Could you check a few things on this model? Use its own coordinates, in mm. Face numbers are marked on the shaded views. A direction names the side the tool comes from. Round coordinates to 2 decimals unless told otherwise and drop trailing zeros. Loops run counter-clockwise (first coordinate to the right, second up) from the corner with the lowest first, then second, coordinate; pieces in that order, holes last. Notation, with made-up numbers: (64.25, 46.25) - (87.25, 46.25) arc R17 ccw to (87.25, 61.25) - close; hole circle Ø7 at (2.25, 12.25). An arc over 180 degrees is marked (long way). Use one line per item in the form item = value.
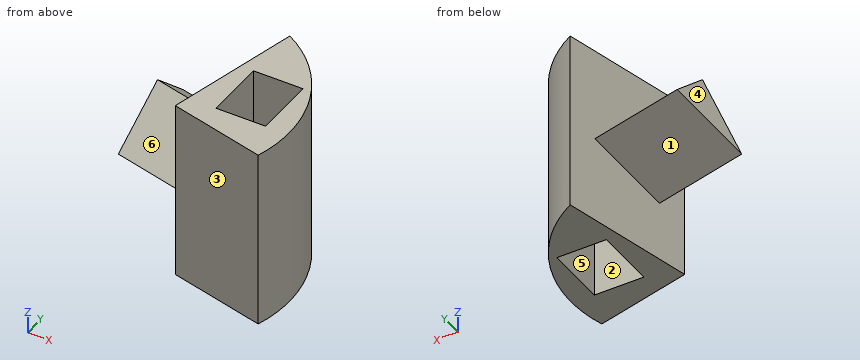
```python
from build123d import *

# Parameters (mm, degrees)
F0_W     = 12.7
F0_H     = 15.9213780425
F1_DEPTH = 46.482
F3_DEPTH = 25.4


with BuildPart() as f1:
    # F0 (on Top) → F1 (new body)
    with BuildSketch(Plane.XY):
        with BuildLine():
            ThreePointArc((16.7416256447, -20.4212910858), (15.8982302722, 2.9417746338), (0.3078590999, 20.3625806509))
            Line((0.3078590999, 20.3625806509), (-8.168171327, -14.3365160608))
            Line((-8.168171327, -14.3365160608), (16.7416256447, -20.4212910858))
        make_face()
        with Locations((6.35, -2.5750233326)):
            Rectangle(F0_W, F0_H, mode=Mode.SUBTRACT)
    extrude(amount=F1_DEPTH)

    # F2 (on face) → F3 (join)
    with BuildSketch(Plane(origin=(-4.40340964, 1.0756312881, 0), x_dir=(-0.2372953486, -0.9714375521, 0), z_dir=(-0.9714375521, 0.2372953486, 0))):
        Polygon((8.0335900158, 15.4112059095), (-4.2063454166, 29.3332058936), (-12.0916292071, 22.4006269127), align=None)
    extrude(amount=F3_DEPTH)


solid = f1.part
```
1. Please list where these lines run through material, in increasing order: line 1 along Y through (x, z) = (7.5, 20.5); line 2 along X through (y, z) = (3, 4); line 3 along X through (y, z) = (-3, 37).
Solution:
line_1 = -18.16 to -10.54, 5.39 to 15.2
line_2 = -3.93 to 0, 12.7 to 15.87
line_3 = -5.4 to 0, 12.7 to 17.69
2. If we section it at C-C, the plane y = 15.5: Write out the boundary of the cut face in (x, z).
Solution:
outline = (-27.03, 21.2) - (-12.5, 22.4) - (-27.03, 25.43) - close; (-0.88, 0) - (7.17, 0) - (7.17, 46.48) - (-0.88, 46.48) - close
3. For P1, Ø5, axis at x = -10, z = 27.5, coming from the +Y side; P2, Ø2, axis at x = -0.5, z = 9.5, coming from the -Y side; P3, Ø6.5, axis at x = 4.5, z = 27, coming from the -Y side, each with a flat end and sliding along its axis, tell me the tip position at first contact or that it passes through.
Solution:
P1 = 11.91
P2 = -16.45
P3 = -18.22
4. On a 3-axis mill with a long thin cutter (end or side, diameter ignored), from which of +Z, -Z, +X, -X, +Y, -Y can I reach the whole of each face in a straight line? I mean the marked faces 4, 5 and 6. Say none if no direction works.
Solution:
face_4 = +Z, -Z, -X, +Y
face_5 = +Z, -Z
face_6 = +Z, -X
5. If we section it at A-A, the plane z = 7: Write out the boundary of the cut face in (x, y).
Solution:
outline = (-8.17, -14.34) - (16.74, -20.42) arc R34.38 ccw to (0.31, 20.36) - close; hole (0, -10.54) - (12.7, -10.54) - (12.7, 5.39) - (0, 5.39) - close
6. If we section it at B-B, the plane x = 10: Write out the boundary of the cut face in (y, z), plus the area to 3 significant figures.
Solution:
outline = (-18.77, 0) - (-10.54, 0) - (-10.54, 46.48) - (-18.77, 46.48) - close; (5.39, 0) - (12.6, 0) - (12.6, 46.48) - (5.39, 46.48) - close
area = 718 mm^2
7. We'd pull the mould along Y, two halves only. Please class the marked faces 1, 2 and 3: +Y half, -Y half, draft (parallel to the pull), parting line (faces both ways), or undercut.
Solution:
face_1 = +Y half
face_2 = undercut
face_3 = -Y half
8. If we section it at D-D, the plane y = 7.5: Write out the boundary of the cut face in (x, z), plus the area to 3 significant figures.
Solution:
outline = (-28.98, 18.34) - (-2.83, 20.5) - (-2.83, 0) - (13.66, 0) - (13.66, 46.48) - (-2.83, 46.48) - (-2.83, 27.22) - (-12.98, 29.33) - (-28.98, 25.01) - close
area = 980 mm^2
